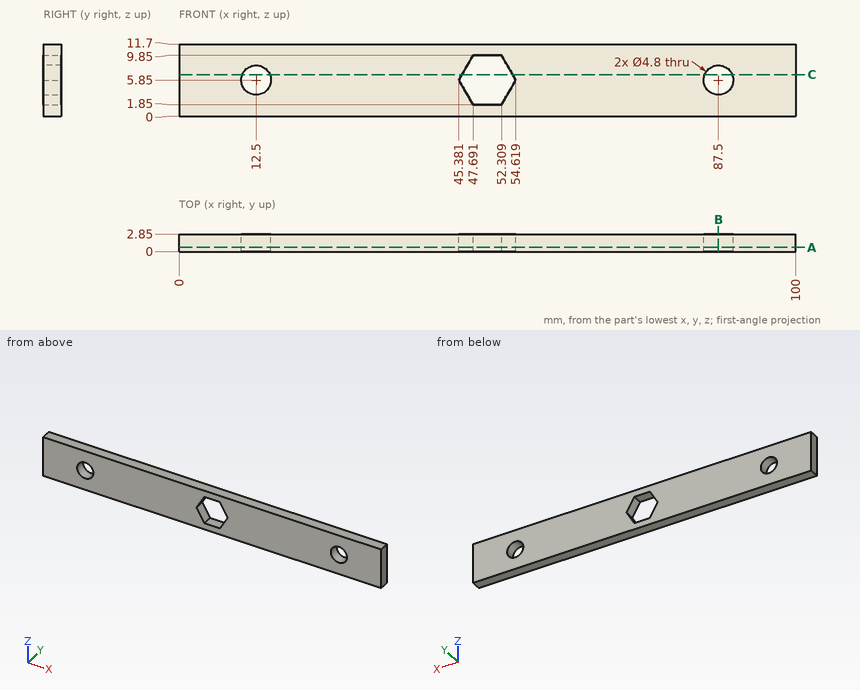
Here's the drawing with two shaded views (mm, measured from the low corner). I have some questions. Coordinates: 2 decimals unless noted, no trailing zeros. Loops run counter-clockwise (first coordinate to the right, second up) from the corner with the lowest first, then second, coordinate; pieces in that order, holes last. Notation, with made-up numbers: M 29,39 L 77,39 A25 cw 77,67 Z; hole C 88.5,25.5 d5. An arc over 180 degrees is marked long. Return JSON: item names as keys, results as strings. Group by question number.
Item 1: If I drill on L1, parallel to X at y = 0.6, z = 5.85; L2, parallel to X at y = 2.2, z = 6 (1 decimal); L3, parallel to Z at x = 48.5, y = 2.55, over which ranges is the centre line in solid material (lowest first)? Write a range as from..to.
Item 2: Imagine slicing it at B-B (x = 87.5). Please give me the cut outline in (y, z).
Item 3: Imagine slicing it at C-C (z = 6.75). Give the number of separate pieces and of enclosed holes in the cut face, and give its area (3 significant figures).
Item 4: I'm going to push a flat-ended pin straight in: pin 1 Ø5.5 at (x, z) = (12.5, 5.85) entering from -Y. Where does the tip first touch, or does it pass through?
Item 5: Imagine slicing it at A-A (y = 0.7). Please give me the cut outline in (x, z), and give its area (3 significant figures).
Verdict:
{
 "1": {"L1": "x = 0..10.1, 14.9..45.38, 54.62..85.1, 89.9..100", "L2": "x = 0..10.1, 14.9..45.5, 54.5..85.1, 89.9..100", "L3": "z = 0..1.85, 9.85..11.7"},
 "2": {"outline": "M 0,0 L 2.85,0 L 2.85,3.45 L 0,3.45 Z; M 0,8.25 L 2.85,8.25 L 2.85,11.7 L 0,11.7 Z"},
 "3": {"separate pieces": "4", "enclosed holes": "0", "area": "236 mm^2"},
 "4": {"pin 1": "stops at y = 0"},
 "5": {"outline": "M 0,0 L 100,0 L 100,11.7 L 0,11.7 Z; hole C 12.5,5.85 d4.8; hole M 45.38,5.85 L 47.69,1.85 L 52.31,1.85 L 54.62,5.85 L 52.31,9.85 L 47.69,9.85 Z; hole C 87.5,5.85 d4.8", "area": "1,080 mm^2"}
}
